CAD build for the part. Positions are in the model's coordinates, mm. A direction names the side the tool comes from. Coordinates: 2 decimals unless noted, no trailing zeros. Write each loop counter-clockwise with the first axis right and the second up, starting at its lowest first coordinate (ties: lowest second). Pieces come first, ordered by that corner, then holes. Notation, with made-up numbers: (23, 85) -> (76, 85) arc R19 cw to (76, 89) -> close; hole circle Ø6 at (25, 19). An arc over 180 degrees is marked (long way). Answer as CSV lines item,"result".
```python
from build123d import *

# Parameters (mm, degrees)
SKETCH_2_R               = 1.2
CUT_EXTRUDE_1_DEPTH      = 10
PATTERN_CIRCULAR_1_COUNT = 12


with BuildPart() as part:
    # 草图1 → 旋转1 (revolve)
    with BuildSketch(Plane.XY):
        Polygon((-53, 0), (-59, 0), (-59, 10), (-51.2, 10), (-51.2, 8), (-53, 8), align=None)
    revolve(axis=Axis((0, 0, 0), (0, 1, 0)))

    # 草图2 → 切除-拉伸1 (cut)
    with BuildSketch(Plane.XZ):
        with Locations((0, 56)):
            Circle(SKETCH_2_R)
    cut_extrude_1 = extrude(amount=-CUT_EXTRUDE_1_DEPTH, mode=Mode.SUBTRACT)

    # 阵列(圆周)1: 切除-拉伸1 ×12 about axis
    pattern_circular_1_axis = Axis((0, 0, 0), (0, 1, 0))
    for i in range(1, PATTERN_CIRCULAR_1_COUNT):
        add(cut_extrude_1.rotate(pattern_circular_1_axis, i * 360 / PATTERN_CIRCULAR_1_COUNT), mode=Mode.SUBTRACT)


solid = part.part
```
Item 1: Flat gauge pins, fed straight in: pin 1 (3 mm diameter, centred on y = 5.5, z = 31.5, fed in from -X); pin 2 (4 mm diameter, centred on x = 28, z = -48.5, fed in from -Y); pin 3 (4 mm diameter, centred on y = 8, z = 21, fed in from -X); pin 4 (2 mm diameter, centred on x = 31, y = 9, fed in from -Z). Where does each tip first touch, or does it go through?
Answer below:
pin 1,"stops at x = -50.8"
pin 2,"stops at y = 0"
pin 3,"stops at x = -55.86"
pin 4,"stops at z = -50.8"
Item 2: Wall check: line 1 (Z direction, x = 0, y = 7); line 2 (Z direction, x = 49, y = 1); line 3 (X direction, y = 4.75, z = 42.5). Give the ranges that are in metal, low to high. Write a range as from..to.
Answer below:
line 1,"z = -59..-57.2, -54.8..-53, 53..54.8, 57.2..59"
line 2,"z = -32.86..-29.09, -26.91..-20.2, 20.2..26.91, 29.09..32.86"
line 3,"x = -40.92..-31.67, 31.67..40.92"
Item 3: 3-axis set-ups, long thin cutter, end or side, ignore diameter. For faces 4 (the flat face through (-27.7, 8, 43.4)), 5 (the cylindrical face through (40.631, 8.986, -31.154)): which of +Z, -Z, +X, -X, +Y, -Y reach the whole face in a straight line?
Answer below:
face 4,"-Y"
face 5,"+Y, -Y"
Item 4: Saw through at A-A on z = 43. Give the cut face in (x, y), and give its area (3 significant figures).
Answer below:
outline,"(-40.4, 0) -> (-30.98, 0) -> (-30.98, 8) -> (-27.79, 8) -> (-27.79, 10) -> (-40.4, 10) -> close; (27.79, 8) -> (30.98, 8) -> (30.98, 0) -> (40.4, 0) -> (40.4, 10) -> (27.79, 10) -> close"
area,"201 mm2"
Item 5: Saw through at B-B on x = 43.5. Give the cut face in (y, z), and give its area (3 significant figures).
Answer below:
outline,"(0, -39.86) -> (10, -39.86) -> (10, -27) -> (8, -27) -> (8, -30.28) -> (0, -30.28) -> close; (0, 30.28) -> (8, 30.28) -> (8, 27) -> (10, 27) -> (10, 39.86) -> (0, 39.86) -> close"
area,"205 mm2"
Item 6: Saw through at C-C on y = 3. State how many separate pieces and enclosed holes the cut face has, and give its area (3 significant figures).
Answer below:
separate pieces,"1"
enclosed holes,"13"
area,"2,060 mm2"
Item 7: Two-plate mould, pull along Z, no slides. Class faces 1 (the flat face through (-22.13, 0, 48.35)), 2 (the cylindrical face through (-28, 4, 45)), 3 (the cylindrical face through (-56.275, 5.07, 17.722)): pulls with the +Z half, pulls with the -Z half, needs draft (parallel to the pull), parting line crosses it, or undercut.
Answer below:
face 1,"needs draft"
face 2,"undercut"
face 3,"parting line crosses it"
